```python
from build123d import *

# Parameters (mm, degrees)
SKETCH1_W           = 10
SKETCH1_H           = 114.68
BOSS_EXTRUDE1_DEPTH = 5
BOSS_EXTRUDE2_DEPTH = 10


with BuildPart() as part:
    # Sketch1 → Boss-Extrude1 (new body)
    with BuildSketch(Plane(origin=(0, 0, 0), x_dir=(1, 0, 0), z_dir=(0, 1, 0))):
        with Locations((5, 57.34)):
            Rectangle(SKETCH1_W, SKETCH1_H)
    extrude(amount=BOSS_EXTRUDE1_DEPTH)

    # Sketch3 → Boss-Extrude2 (add, through all)
    with BuildSketch(Plane(origin=(10, 0, 0), x_dir=(0, 0, -1), z_dir=(1, 0, 0))):
        Polygon((0.75, 9.1), (0, 9.1), (0, 0), (-2.5, 0), (-2.5, 9.1), (-2.5, 11.6), (0.75, 11.6), align=None)
        Polygon((114.68, 0), (117.18, 0), (117.18, 14.6), (117.18, 17.1), (113.93, 17.1), (113.93, 14.6), (114.68, 14.6), align=None)
    extrude(amount=-BOSS_EXTRUDE2_DEPTH)


solid = part.part
```
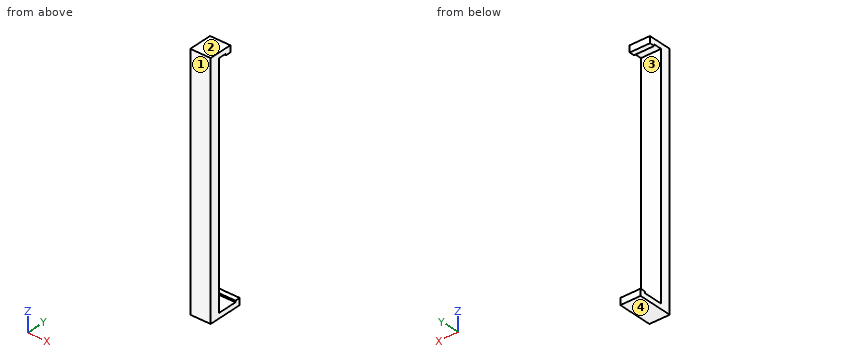
Can you work these out from the model? Positions are in its coordinate system, mm. Face numbers are marked on the shaded views. Round coordinates to 2 decimals unless told otherwise and drop trailing zeros. Loops run counter-clockwise (first coordinate to the right, second up) from the corner with the lowest first, then second, coordinate; pieces in that order, holes last.
Item 1: Please list where these lines run through material, in increasing order: L1, parallel to Z at x = 4, y = 9.25; L2, parallel to Z at x = 4, y = 7.75; L3, parallel to Y at x = 6.5, z = -49.5.
Item 2: If we mould it in two halves opening along Z, with no side actions, what happens to the marked faces 1, 2, 3 and 4? For each: +Z half, -Z half, draft (parallel to the pull), parting line (faces both ways), or undercut.
Item 3: Suppose I cut it at B-B, the plane x = 8. Write out the boundary of the cut face in (y, z).
Item 4: Suppose I cut it at C-C, the plane z = -47. Write out the boundary of the cut face in (x, y).
Item 5: Suppose I cut it at A-A, the plane y = 7. Write out the boundary of the cut face in (x, z), then the cut area to 3 significant figures.
Item 6: Will these pins go through, and if not, where does the flat tip stop? pin 1 Ø5 at (x, z) = (5.5, -76.5) entering from +Y; pin 2 Ø10 at (y, z) = (7, -10.5) entering from +X; pin 3 Ø1.6 at (x, z) = (5.5, 1.5) entering from +Y; pin 4 Ø3 at (x, y) = (7.5, 16) entering from +Z.
Reported:
1. L1: z = -117.18 to -114.68, -0.75 to 2.5
1. L2: z = -117.18 to -114.68, 0 to 2.5
1. L3: y = 0 to 5
2. face 1: draft
2. face 2: +Z half
2. face 3: undercut
2. face 4: -Z half
3. outline: (0, -117.18) - (17.1, -117.18) - (17.1, -113.93) - (14.6, -113.93) - (14.6, -114.68) - (5, -114.68) - (5, 0) - (9.1, 0) - (9.1, -0.75) - (11.6, -0.75) - (11.6, 2.5) - (0, 2.5) - close
4. outline: (0, 0) - (10, 0) - (10, 5) - (0, 5) - close
5. outline: (0, -117.18) - (10, -117.18) - (10, -114.68) - (0, -114.68) - close; (0, 0) - (10, 0) - (10, 2.5) - (0, 2.5) - close
5. area: 50.0 mm2
6. pin 1: stops at y = 5
6. pin 2: stops at x = 10
6. pin 3: stops at y = 11.6
6. pin 4: stops at z = -113.93
